The listing builds one solid part. Answer for the finished solid, in the listing's coordinates (mm). A direction names the side the tool comes from. Coordinates: 2 decimals unless noted, no trailing zeros. Write each loop counter-clockwise with the first axis right and the second up, starting at its lowest first coordinate (ties: lowest second). Pieces come first, ordered by that corner, then holes.
from build123d import *

# Parameters (mm, degrees)
SKETCH1_W           = 28
SKETCH1_H           = 33.5
BOSS_EXTRUDE1_DEPTH = 22
CUT_EXTRUDE1_DEPTH  = 44
SKETCH4_W           = 10
SKETCH4_H           = 2
CUT_EXTRUDE3_DEPTH  = 49


with BuildPart() as part:
    # Sketch1 → Boss-Extrude1 (new body)
    with BuildSketch(Plane(origin=(0, 0, 0), x_dir=(1, 0, 0), z_dir=(0, 1, 0))):
        Rectangle(SKETCH1_W, SKETCH1_H)
    extrude(amount=BOSS_EXTRUDE1_DEPTH)

    # Sketch3 → Cut-Extrude1 (cut)
    with BuildSketch(Plane.XY.offset(16.75)):
        Polygon((14, 22), (-14, 22), (14, 3), align=None)
    extrude(amount=-CUT_EXTRUDE1_DEPTH, mode=Mode.SUBTRACT)

    # Sketch4 → Cut-Extrude3 (cut)
    with BuildSketch(Plane.XZ):
        with Locations((-9, 15.75)):
            Rectangle(SKETCH4_W, SKETCH4_H)
        with Locations((-9, -15.75)):
            Rectangle(SKETCH4_W, SKETCH4_H)
    extrude(amount=-CUT_EXTRUDE3_DEPTH, mode=Mode.SUBTRACT)


solid = part.part
1. Flat-ended cylindrical pins translate along their axes: P1, Ø10, axis at x = 5.5, z = -9, coming from the +Y side; P2, Ø1.5, axis at x = -9.5, y = 7.5, coming from the +Z side; P3, Ø1, axis at y = 7, z = -16, coming from the -X side. Find the tip coordinate at first contact, or state that the pin passes through.
Results found:
P1: stops at y = 12.16
P2: stops at z = 14.75
P3: stops at x = -4
2. Section B-B on z = -2 is taken. Give the vertices of the cut face in (x, y).
Results found:
outline: (-14, 0) - (14, 0) - (14, 3) - (-14, 22) - close
3. Find the intervals of material crossed by L1, parallel to Z at x = -10, y = 10; L2, parallel to Y at x = 1.5, z = -12.5; L3, parallel to Y at x = -6.75, z = -10, in increasing order.
Results found:
L1: z = -14.75 to 14.75
L2: y = 0 to 11.48
L3: y = 0 to 17.08
4. Section C-C on x = 3.75 is taken. Give the vertices of the cut face in (y, z).
Results found:
outline: (0, -16.75) - (9.96, -16.75) - (9.96, 16.75) - (0, 16.75) - close
5. Section D-D on y = 8.5 is taken. Give the vertices of the cut face in (x, z), then the cut area to 3 significant figures.
Results found:
outline: (-14, -14.75) - (-4, -14.75) - (-4, -16.75) - (5.89, -16.75) - (5.89, 16.75) - (-4, 16.75) - (-4, 14.75) - (-14, 14.75) - close
area: 626 mm2
6. Section A-A on y = 5.25 is taken. Give the vertices of the cut face in (x, z).
Results found:
outline: (-14, -14.75) - (-4, -14.75) - (-4, -16.75) - (10.68, -16.75) - (10.68, 16.75) - (-4, 16.75) - (-4, 14.75) - (-14, 14.75) - close
7. A tool of negligible diameter and unlimited length cuts with its end or side. For faces 1 (the flat face through (-9, 8, 14.75)), 2 (the flat face through (-0.196, 12.633, 0.235)), 3 (the flat face through (-9, 8, -14.75)), from which of +Z, -Z, +X, -X, +Y, -Y can it reach the whole face along a straight path? Write none if from no direction.
Results found:
face 1: +Z, -X, +Y, -Y
face 2: +Z, -Z, +X, +Y
face 3: -Z, -X, +Y, -Y
